from build123d import *

# Parameters (mm, degrees)
F1_DEPTH = 700


with BuildPart() as f1:
    # F0 (on Front) → F1 (new body)
    with BuildSketch(Plane.XZ):
        with BuildLine():
            Line((8, -20), (20, -20))
            Line((20, -20), (20, -8))
            ThreePointArc((20, -8), (12, 0), (20, 8))
            Line((20, 8), (20, 20))
            Line((20, 20), (8, 20))
            ThreePointArc((8, 20), (0, 12), (-8, 20))
            Line((-8, 20), (-20, 20))
            Line((-20, 20), (-20, 8))
            ThreePointArc((-20, 8), (-14.343146, 5.656854), (-12, 0))
            ThreePointArc((-12, 0), (-14.343146, -5.656854), (-20, -8))
            Line((-20, -8), (-20, -20))
            Line((-20, -20), (-8, -20))
            ThreePointArc((-8, -20), (0, -12), (8, -20))
        make_face()
    extrude(amount=F1_DEPTH)


solid = f1.part
Here's how the part is built. I have some questions about the finished solid (model axes, mm). Coordinates: 2 decimals unless noted, no trailing zeros. Write each loop counter-clockwise with the first axis right and the second up, starting at its lowest first coordinate (ties: lowest second). Pieces come first, ordered by that corner, then holes.
Item 1: If we mould it in two halves opening along X, with no side actions, what happens to faces 1 (the cylindrical face through (0, -345, -12)), 2 (the cylindrical face through (0, -345, 12)), 3 (the flat face through (-20, -345, -14)), 4 (the flat face through (14, -345, 20))? For each: +X half, -X half, draft (parallel to the pull), parting line (faces both ways), or undercut.
Item 2: I want a section at B-B on x = 0. Write out the boundary of the cut face in (y, z).
Item 3: Will this pin go through, and if not, where does the flat tip stop? pin 1 (12 mm diameter, centred on x = 0.5, y = -75, fed in from -Z).
Item 4: If I drill on line 1 (Z direction, x = -14.5, y = -521); line 2 (X direction, y = -420, z = -0.5); line 3 (Z direction, x = 1, y = -536), over which ranges is the centre line in solid material (lowest first)?
Item 5: I want a section at A-A on y = -629.5. Write out the boundary of the cut face in (x, z), and give its area (3 significant figures).
Findings below:
1. face 1: undercut
1. face 2: undercut
1. face 3: -X half
1. face 4: draft
2. outline: (-700, -12) - (0, -12) - (0, 12) - (-700, 12) - close
3. pin 1: stops at z = -15.34
4. line 1: z = -20 to -5.81, 5.81 to 20
4. line 2: x = -12.02 to 12.02
4. line 3: z = -12.06 to 12.06
5. outline: (-20, -20) - (-8, -20) arc R8 cw to (8, -20) - (20, -20) - (20, -8) arc R8 cw to (20, 8) - (20, 20) - (8, 20) arc R8 cw to (-8, 20) - (-20, 20) - (-20, 8) arc R8 cw to (-12, 0) arc R8 cw to (-20, -8) - close
5. area: 1,200 mm2
